Autodesk Inventor part; units mm, degrees
ref_plane "YZ Plane" through (0, 0, 0) normal (1, 0, 0) x (0, 1, 0)
ref_plane "XZ Plane" through (0, 0, 0) normal (0, 1, 0) x (-1, 0, 0)
ref_plane "XY Plane" through (0, 0, 0) normal (0, 0, 1) x (1, 0, 0)
sketch "Эскиз1" plane through (0, 0, 0) normal (0, 0, 1) x (1, 0, 0)
  circle A0 centre (0, 0) radius 44
  circle A1 centre (-45.8993, 26.5) radius 5
  circle A2 centre (45.8993, 26.5) radius 5
  circle A3 centre (0, -53) radius 5
  line L0 (0, 0) -> (-45.8993, 26.5) construction
  line L1 (0, 0) -> (45.8993, 26.5) construction
  line L2 (0, -53) -> (0, 0) construction
  arc A4 (-51.6909, 11.7068) -> (-53.6716, 20.2078) centre (-61.4439, 13.9156) ccw
  arc A5 (-44.3363, 36.3771) -> (-53.6716, 20.2078) centre (-45.8993, 26.5) ccw
  arc A6 (-44.3363, 36.3771) -> (-35.9838, 38.9122) centre (-42.7733, 46.2542) ccw
  arc A7 (35.9838, 38.9122) -> (44.3363, 36.3771) centre (42.7733, 46.2542) ccw
  arc A8 (53.6716, 20.2078) -> (44.3363, 36.3771) centre (45.8993, 26.5) ccw
  arc A9 (53.6716, 20.2078) -> (51.6909, 11.7068) centre (61.4439, 13.9156) ccw
  arc A10 (15.7071, -50.619) -> (9.3353, -56.5849) centre (18.6707, -60.1698) ccw
  arc A11 (-9.3353, -56.5849) -> (9.3353, -56.5849) centre (0, -53) ccw
  arc A12 (-9.3353, -56.5849) -> (-15.7071, -50.619) centre (-18.6707, -60.1698) ccw
  arc A13 (4.9944, -52.7642) -> (0, -53) centre (0, 0) ccw construction
  arc A14 (35.9838, 38.9122) -> (-35.9838, 38.9122) centre (0, 0) ccw
  arc A15 (-51.6909, 11.7068) -> (-15.7071, -50.619) centre (0, 0) ccw
  arc A16 (15.7071, -50.619) -> (51.6909, 11.7068) centre (0, 0) ccw
  dimension "d0" = 88
  dimension "d2" = 10
  dimension "d3" = 120
  dimension "d4" = 120
  dimension "d6" = 10
  dimension "d7" = 106
  dimension "d8" = 53
  dimension "d10" = 53
extrude "Выдавливание1" add sketch "Эскиз1" along normal mid plane 1
properties part number "79. Прокладка"
Source: CAD feature listing. Evaluate the final solid. Frame: model axes, mm. Round coordinates to 2 decimals unless told otherwise and drop trailing zeros. Write each loop counter-clockwise with the first axis right and the second up, starting at its lowest first coordinate (ties: lowest second). Pieces come first, ordered by that corner, then holes. Notation, with made-up numbers: M 30,55 L 39,55 A20 ccw 39,90 Z; hole C 84.5,48 d10. An arc over 180 degrees is marked long. Use CSV: the item, a comma, the result in double quotes. Start each with the question number.
Q1. Cut plane C-C on y = 26.5. Output: boundary loops of the cut face in (x, z), plus the area to 3 significant figures.
Q2. Cut plane A-A on y = 0. Output: boundary loops of the cut face in (x, z), plus the area to 3 significant figures.
Q3. Line query: line 1 (X direction, y = -1, z = -0.4); line 2 (X direction, y = 30, z = -0.2); line 3 (X direction, y = -39, z = -0.2). Output: solid intervals per line, ascending. Write a range as from..to.
Q4. Cut plane D-D on x = 0. Output: boundary loops of the cut face in (y, z), plus the area to 3 significant figures.
Q5. First-contact query: P1, Ø6, axis at x = 0, y = -53, coming from the +Z side. Flat tip, straight axial feed; report the tip coordinate or a pass-through.
Q6. Pull-direction query (Y, two-part tool) for faces 1 (the face through (54.5, 31.6, 0)), 2 (the face through (-8.5, -43.4, 0.5)), 3 (the face through (39.929, 36.667, -0.007)), 4 (the face through (41.9, 29.5, 0)); classes: +Y half, -Y half, draft (parallel to the pull), parting line (faces both ways), or undercut.
Q7. Cut plane B-B on x = -39.5. Output: boundary loops of the cut face in (y, z).
Results found:
1,outline,"M -55.9,-0.5 L -50.9,-0.5 L -50.9,0.5 L -55.9,0.5 Z; M -40.9,-0.5 L -35.12,-0.5 L -35.12,0.5 L -40.9,0.5 Z; M 35.12,-0.5 L 40.9,-0.5 L 40.9,0.5 L 35.12,0.5 Z; M 50.9,-0.5 L 55.9,-0.5 L 55.9,0.5 L 50.9,0.5 Z"
1,area,"21.5 mm^2"
2,outline,"M -53,-0.5 L -44,-0.5 L -44,0.5 L -53,0.5 Z; M 44,-0.5 L 53,-0.5 L 53,0.5 L 44,0.5 Z"
2,area,"18.0 mm^2"
3,line 1,"-52.99..-43.99, 43.99..52.99"
3,line 2,"-55.27..-49.47, -42.33..-32.19, 32.19..42.33, 49.47..55.27"
3,line 3,"-35.89..-20.37, 20.37..35.89"
4,outline,"M -63,-0.5 L -58,-0.5 L -58,0.5 L -63,0.5 Z; M -48,-0.5 L -44,-0.5 L -44,0.5 L -48,0.5 Z; M 44,-0.5 L 53,-0.5 L 53,0.5 L 44,0.5 Z"
4,area,"18.0 mm^2"
5,P1,"through"
6,face 1,"parting line"
6,face 2,"draft"
6,face 3,"+Y half"
6,face 4,"undercut"
7,outline,"M -35.34,-0.5 L -19.38,-0.5 L -19.38,0.5 L -35.34,0.5 Z; M 19.38,-0.5 L 36.81,-0.5 L 36.81,0.5 L 19.38,0.5 Z"
